from build123d import *

# Parameters (mm, degrees)
BASE_SKETCH_W    = 31.8
BASE_SKETCH_H    = 7.8
BASE_BRICK_DEPTH = 3.2
CIRCLE_SKETCH_R  = 2.4
CIRCLE_DEPTH     = 1.7
LPATTERN1_COUNT  = 4
LPATTERN1_PITCH  = 8


with BuildPart() as part:
    # Base_Sketch → Base_Brick (new body)
    with BuildSketch(Plane(origin=(0, 0, 0), x_dir=(1, 0, 0), z_dir=(0, 1, 0))):
        with Locations((15.9, 3.9)):
            Rectangle(BASE_SKETCH_W, BASE_SKETCH_H)
    extrude(amount=BASE_BRICK_DEPTH)

    # Circle_Sketch → Circle (add)
    with BuildSketch(Plane(origin=(0, 3.2, 0), x_dir=(1, 0, 0), z_dir=(0, 1, 0))):
        with Locations(Location((3.9, 3.9, 0), (0, 0, 90))):
            Circle(CIRCLE_SKETCH_R)
    circle = extrude(amount=CIRCLE_DEPTH)

    # LPattern1: Circle ×4
    with Locations(*[(i * LPATTERN1_PITCH, 0, 0) for i in range(1, LPATTERN1_COUNT)]):
        add(circle)


solid = part.part
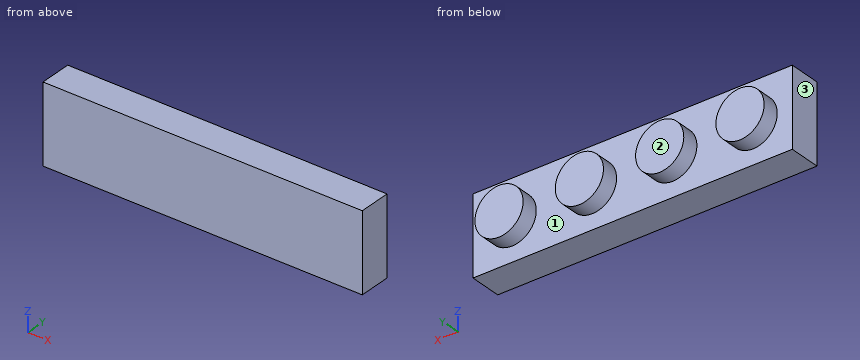
Source: CAD feature listing. Evaluate the final solid. Frame: model axes, mm. Face numbers are marked on the shaded views. Give positions to 0.01 mm unless a question says otherwise; leave off trailing zeros. Order: outer loops, then holes, each group sorted by start corner. A loop starts at its lowest first (then second) coordinate and runs counter-clockwise, first axis right, second up. Notation, with made-up numbers: (-15.5, -25) -> (-3.5, -25) arc R22 ccw to (-3.5, -3) -> close; hole circle Ø1 at (45, -19). An arc over 180 degrees is marked (long way). Write item = value, one per line.
Item 1: Section query A-A (y = 4.3). Output: boundary loops of the cut face in (x, z), then the cut area to 3 significant figures.
Check result:
outline = circle Ø4.8 at (3.9, -3.9); circle Ø4.8 at (11.9, -3.9); circle Ø4.8 at (19.9, -3.9); circle Ø4.8 at (27.9, -3.9)
area = 72.4 mm²
Item 2: Section query D-D (x = 19.9). Output: boundary loops of the cut face in (y, z), then the cut area to 3 significant figures.
Check result:
outline = (0, -7.8) -> (3.2, -7.8) -> (3.2, -6.3) -> (4.9, -6.3) -> (4.9, -1.5) -> (3.2, -1.5) -> (3.2, 0) -> (0, 0) -> close
area = 33.1 mm²
Item 3: Ray query, probe 1 along X at (y, z) = (3.3, -1.75); probe 2 along Y at (x, z) = (13.5, -0.75); probe 3 along X at (y, z) = (3.6, -2.5). Return the intervals inside material, ascending.
Check result:
probe_1 = 2.83 to 4.97, 10.83 to 12.97, 18.83 to 20.97, 26.83 to 28.97
probe_2 = 0 to 3.2
probe_3 = 1.95 to 5.85, 9.95 to 13.85, 17.95 to 21.85, 25.95 to 29.85
Item 4: Section query B-B (z = -3.9). Output: boundary loops of the cut face in (x, y), then the cut area to 3 significant figures.
Check result:
outline = (0, 0) -> (31.8, 0) -> (31.8, 3.2) -> (30.3, 3.2) -> (30.3, 4.9) -> (25.5, 4.9) -> (25.5, 3.2) -> (22.3, 3.2) -> (22.3, 4.9) -> (17.5, 4.9) -> (17.5, 3.2) -> (14.3, 3.2) -> (14.3, 4.9) -> (9.5, 4.9) -> (9.5, 3.2) -> (6.3, 3.2) -> (6.3, 4.9) -> (1.5, 4.9) -> (1.5, 3.2) -> (0, 3.2) -> close
area = 134 mm²
Item 5: Section query C-C (x = 3.5). Output: boundary loops of the cut face in (y, z), then the cut area to 3 significant figures.
Check result:
outline = (0, -7.8) -> (3.2, -7.8) -> (3.2, -6.27) -> (4.9, -6.27) -> (4.9, -1.53) -> (3.2, -1.53) -> (3.2, 0) -> (0, 0) -> close
area = 33.0 mm²
Item 6: Mould query, pull axis X, two halves, no side actions, for the marked faces 1, 2 and 3. Classes: +X half, -X half, draft (parallel to the pull), parting line (faces both ways), or undercut.
Check result:
face_1 = undercut
face_2 = draft
face_3 = -X half
